```python
from build123d import *

# Parameters (mm, degrees)
EXTRUDE_1_DEPTH = 8
SKETCH_2_R      = 6
EXTRUDE_2_DEPTH = 80
CHAMFER_1_SIZE  = 2
CHAMFER_1_SIZE2 = 1.154700538


with BuildPart() as part:
    # Эскиз1 → Бобышка-Вытянуть1 (new body)
    with BuildSketch(Plane(origin=(0, 0, 0), x_dir=(1, 0, 0), z_dir=(0, 1, 0))):
        Polygon((9.374335606, -5.696943503), (9.620865601, 5.269941027), (0.246529995, 10.96688453), (-9.374335606, 5.696943503), (-9.620865601, -5.269941027), (-0.246529995, -10.96688453), align=None)
    extrude(amount=EXTRUDE_1_DEPTH)

    # Эскиз2 → Бобышка-Вытянуть2 (add)
    with BuildSketch(Plane(origin=(0, 8, 0), x_dir=(1, 0, 0), z_dir=(0, 1, 0))):
        Circle(SKETCH_2_R)
    extrude(amount=EXTRUDE_2_DEPTH)

    # Фаска1
    chamfer_1_edges = [part.edges().sort_by_distance(p)[0] for p in [
        (-4.933697798, 0, 8.118412778),
        (-9.497600603, 0, -0.213501238),
        (-4.563902806, 0, -8.331914017),
        (4.933697798, 0, -8.118412778),
        (9.497600603, 0, 0.213501238),
        (4.563902806, 0, 8.331914017),
    ]]
    chamfer_1_side = [part.faces().sort_by_distance(p)[0] for p in [
        (0, 0, 0),
    ]]
    chamfer(chamfer_1_edges, length=CHAMFER_1_SIZE, length2=CHAMFER_1_SIZE2, reference=chamfer_1_side[0])


solid = part.part
```
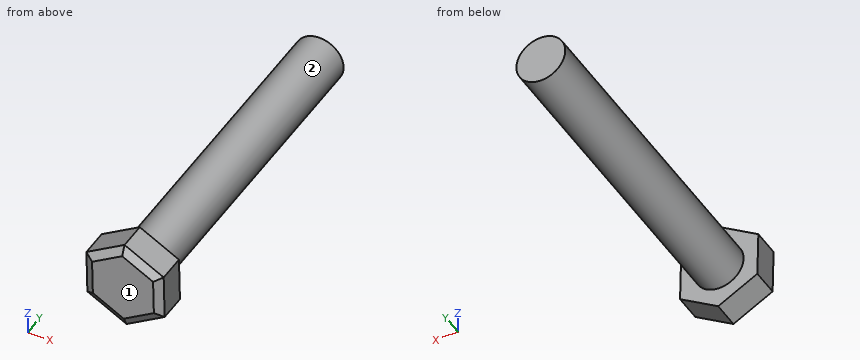
Part model, mm, in its own coordinate system. Face numbers are marked on the shaded views. A direction names the side the tool comes from. Give positions to 0.01 mm unless a question says otherwise; leave off trailing zeros. Order: outer loops, then holes, each group sorted by start corner. A loop starts at its lowest first (then second) coordinate and runs counter-clockwise, first axis right, second up. Notation, with made-up numbers: M 75,75 L 114,75 A15 ccw 114,85 Z; hole C -0.5,-16.5 d5. An arc over 180 degrees is marked long. Use a Markdown table: item, result. Add a question column.
(1) Saw through at D-D, the plane z = -6.75. Give the cut face in (x, y), and give its area (3 significant figures).
(2) Saw through at A-A, the plane x = 1.75. Give the cut face in (y, z), and give its area (4 significant figures).
(3) Saw through at C-C, the plane y = 34. Give the cut face in (x, z), and give its area (3 significant figures).
(4) Drop flat-ended pins along their axis: P1, Ø4, axis at y = 71.5, z = -0.5, coming from the +X side; P2, Ø5, axis at x = 5, y = 61.5, coming from the +Z side; P3, Ø4, axis at y = 29.5, z = 4, coming from the -X side. Give the stop position or say it passes through.
(5) Probe line 1 along Y through (x, z) = (5, 5.5); line 2 along Z through (x, y) = (-0.25, 59.5); line 3 along X through (y, z) = (11, -0.75). List the from-to ranges inside material, lowest first. Write a range as [from, to].
(6) Saw through at B-B, the plane z = 0. Give the cut face in (x, y), and give its area (3 significant figures).
(7) 3-axis set-ups, long thin cutter, end or side, ignore diameter. For the marked faces 1 and 2: which of +Z, -Z, +X, -X, +Y, -Y reach the whole face in a straight line?
Answer key:
| question | item | result |
|---|---|---|
| 1 | outline | M -7.45,1.15 L -3.29,0 L 3.33,0 L 7.19,1.15 L 7.19,8 L -7.45,8 Z |
| 1 | area | 112 mm^2 |
| 2 | outline | M 0,-7.71 L 1.15,-10.05 L 8,-10.05 L 8,-5.74 L 88,-5.74 L 88,5.74 L 8,5.74 L 8,9.87 L 1.15,9.87 L 0,7.59 Z |
| 2 | area | 1,075 mm^2 |
| 3 | outline | C 0,0 d12 |
| 3 | area | 113 mm^2 |
| 4 | P1 | x = 6 |
| 4 | P2 | z = 5.45 |
| 4 | P3 | x = -5.66 |
| 5 | line 1 | [0, 8] |
| 5 | line 2 | [-5.99, 5.99] |
| 5 | line 3 | [-5.95, 5.95] |
| 6 | outline | M -9.5,1.15 L -7.5,0 L 7.5,0 L 9.5,1.15 L 9.5,8 L 6,8 L 6,88 L -6,88 L -6,8 L -9.5,8 Z |
| 6 | area | 1,110 mm^2 |
| 7 | face 1 | +Z, -Z, +X, -X, -Y |
| 7 | face 2 | +Y |
